from build123d import *

# Parameters (mm, degrees)
SKETCH1_W           = 52.1
SKETCH1_H           = 22.8
BOSS_EXTRUDE1_DEPTH = 7.6962
SKETCH2_R           = 2.5
BOSS_EXTRUDE2_DEPTH = 11.2268
SKETCH3_R           = 1.25
CUT_EXTRUDE1_DEPTH  = 19.923


with BuildPart() as part:
    # Sketch1 → Boss-Extrude1 (new body)
    with BuildSketch(Plane(origin=(0, 0, 0), x_dir=(1, 0, 0), z_dir=(0, 1, 0))):
        with Locations((9.186055138, 0.076057393)):
            Rectangle(SKETCH1_W, SKETCH1_H)
    extrude(amount=BOSS_EXTRUDE1_DEPTH)

    # Sketch2 → Boss-Extrude2 (add)
    with BuildSketch(Plane.XZ):
        with Locations((-14.577944862, 8.767742607)):
            Circle(SKETCH2_R)
        with Locations((31.319855138, 8.767742607)):
            Circle(SKETCH2_R)
        with Locations((31.319855138, -9.190057393)):
            Circle(SKETCH2_R)
        with Locations((-14.577944862, -9.190057393)):
            Circle(SKETCH2_R)
    extrude(amount=BOSS_EXTRUDE2_DEPTH)

    # Sketch3 → Cut-Extrude1 (cut, through all)
    with BuildSketch(Plane.XZ.offset(11.2268)):
        with Locations((-14.577944862, 8.767742607)):
            Circle(SKETCH3_R)
        with Locations((-14.577944862, -9.190057393)):
            Circle(SKETCH3_R)
        with Locations((31.319855138, -9.190057393)):
            Circle(SKETCH3_R)
        with Locations((31.319855138, 8.767742607)):
            Circle(SKETCH3_R)
    extrude(amount=-CUT_EXTRUDE1_DEPTH, mode=Mode.SUBTRACT)


solid = part.part
Geometry: final body of the model. Coordinates: model frame, mm. A direction names the side the tool comes from. Round coordinates to 2 decimals unless told otherwise and drop trailing zeros. Write each loop counter-clockwise with the first axis right and the second up, starting at its lowest first coordinate (ties: lowest second). Pieces come first, ordered by that corner, then holes. Notation, with made-up numbers: M 79.5,-0.5 L 130.5,-0.5 A18 cw 130.5,8.5 Z; hole C 8,11 d3. An arc over 180 degrees is marked long. Write item = value, one per line.
Item 1: Section query B-B on x = 23. Return loops of the section in (y, z), then the cut area to 3 significant figures.
Findings:
outline = M 0,-11.48 L 7.7,-11.48 L 7.7,11.32 L 0,11.32 Z
area = 175 mm^2
Item 2: Section query C-C on z = -2.5. Return loops of the section in (x, y), then the cut area to 3 significant figures.
Findings:
outline = M -16.86,0 L 35.24,0 L 35.24,7.7 L -16.86,7.7 Z
area = 401 mm^2
Item 3: Material intervals for line 1 along X through (y, z) = (-6.5, -9.25); line 2 along X through (y, z) = (-7, 9.75); line 3 along X through (y, z) = (0.75, -9.5), sorted ascending. Write a range as [from, to].
Findings:
line_1 = [-17.08, -15.83], [-13.33, -12.08], [28.82, 30.07], [32.57, 33.82]
line_2 = [-16.88, -15.35], [-13.8, -12.28], [29.02, 30.55], [32.09, 33.62]
line_3 = [-16.86, -15.79], [-13.37, 30.11], [32.53, 35.24]
Item 4: Pin query (flat end, axial travel): P1, Ø4, axis at x = -5, z = 2.5, coming from the -Y side; P2, Ø4, axis at x = 9.5, y = 2.5, coming from the -Z side; P3, Ø4, axis at y = 4.5, z = -2, coming from the -X side. Return the tip coordinate at first contact, or that it passes through.
Findings:
P1 = 0
P2 = -11.48
P3 = -16.86
Item 5: Section query A-A on y = -1. Return loops of the section in (x, z), then the cut area to 3 significant figures.
Findings:
outline = C -14.58,-9.19 d5; C -14.58,8.77 d5; C 31.32,-9.19 d5; C 31.32,8.77 d5; hole C -14.58,-9.19 d2.5; hole C -14.58,8.77 d2.5; hole C 31.32,-9.19 d2.5; hole C 31.32,8.77 d2.5
area = 58.9 mm^2
Item 6: Pull-direction query (X, two-part tool) for faces 1 (the face through (-16, -11.227, -10)), 2 (the face through (-15.827, -1.898, 8.823)), 3 (the face through (-16.864, 4, 0)); classes: pulls with the +X half, pulls with the -X half, needs draft (parallel to the pull), parting line crosses it, or undercut.
Findings:
face_1 = needs draft
face_2 = undercut
face_3 = pulls with the -X half
Item 7: Access query for faces 4 (the face through (9, 7.696, 0)), 5 (the face through (-16.5, 0, -11.1)), 6 (the face through (32.66, -5.53, 10.88)). Directions: +Z, -Z, +X, -X, +Y, -Y. A direction counts if a zero-diameter tool reaches every point of the face in a straight line with its end or side. Return the directions, or none.
Findings:
face_4 = +Z, -Z, +X, -X, +Y
face_5 = -Z, -X, -Y
face_6 = -Y
